Here's how the part is built. I have some questions about the finished solid (model axes, mm). Give positions to 0.01 mm unless a question says otherwise; leave off trailing zeros. Order: outer loops, then holes, each group sorted by start corner. A loop starts at its lowest first (then second) coordinate and runs counter-clockwise, first axis right, second up.
from build123d import *

# Parameters (mm, degrees)
BOSS_EXTRUDE1_DEPTH      = 5
BOSS_EXTRUDE1_DEPTH_BACK = 5
BOSS_EXTRUDE2_DEPTH      = 10
CUT_EXTRUDE1_DEPTH       = 262.627597933
SKETCH4_R                = 1.553741305
CUT_EXTRUDE2_DEPTH       = 215.257438611
CHAMFER1_SIZE            = 2
CHAMFER2_SIZE            = 2
FILLET1_R                = 5


with BuildPart() as part:
    # Sketch1 → Boss-Extrude1 (new, two sides: drawn at the far end of the back side and taken through both)
    with BuildSketch(Plane.XY.offset(-BOSS_EXTRUDE1_DEPTH_BACK)):
        Polygon((-87.5, -200), (-87.5, -40), (-50, 0), (50, 0), (87.5, -40), (87.5, -200), (75.5, -200), (75.5, -44.74536976), (44.80121585, -12), (-44.80121585, -12), (-75.5, -44.74536976), (-75.5, -200), align=None)
    extrude(amount=BOSS_EXTRUDE1_DEPTH + BOSS_EXTRUDE1_DEPTH_BACK)

    # Sketch2 → Boss-Extrude2 (add)
    with BuildSketch(Plane.XY.offset(5)):
        Polygon((-87.5, -200), (-75.5, -200), (-75.5, -197), (-75.5, -157), (-80.5, -157), (-80.5, -195), (-87.5, -195), align=None)
    boss_extrude2 = extrude(amount=BOSS_EXTRUDE2_DEPTH)

    # Sketch3 → Cut-Extrude1 (cut, through all)
    with BuildSketch(Plane.ZY.offset(80.5)):
        Polygon((5, -157), (15, -195), (15, -157), align=None)
    cut_extrude1 = extrude(amount=-CUT_EXTRUDE1_DEPTH, mode=Mode.SUBTRACT)

    # Sketch4 → Cut-Extrude2 (cut, through all)
    with BuildSketch(Plane(origin=(0, -195, 0), x_dir=(1, 0, 0), z_dir=(0, 1, 0))):
        with Locations(Location((-84, -10, 0), (0, 0, 270))):
            Circle(SKETCH4_R)
    cut_extrude2 = extrude(amount=-CUT_EXTRUDE2_DEPTH, mode=Mode.SUBTRACT)

    # Mirror1: Boss-Extrude2, Cut-Extrude1, Cut-Extrude2 across plane
    add(boss_extrude2.mirror(Plane(origin=(0, 0, 0), x_dir=(0, 0, 1), z_dir=(1, 0, 0))))
    add(cut_extrude1.mirror(Plane(origin=(0, 0, 0), x_dir=(0, 0, 1), z_dir=(1, 0, 0))), mode=Mode.SUBTRACT)
    add(cut_extrude2.mirror(Plane(origin=(0, 0, 0), x_dir=(0, 0, 1), z_dir=(1, 0, 0))), mode=Mode.SUBTRACT)

    # Chamfer1
    chamfer1_edges = [part.edges().sort_by_distance(p)[0] for p in [
        (-60.150607925, -28.37268488, -5),
        (0, -12, -5),
        (60.150607925, -28.37268488, -5),
        (75.5, -122.37268488, -5),
        (81.5, -200, -5),
        (87.5, -120, -5),
        (68.75, -20, -5),
        (0, 0, -5),
        (-68.75, -20, -5),
        (-87.5, -120, -5),
        (-81.5, -200, -5),
        (-75.5, -122.37268488, -5),
    ]]
    chamfer(chamfer1_edges, length=CHAMFER1_SIZE)

    # Chamfer2
    chamfer2_edges = [part.edges().sort_by_distance(p)[0] for p in [
        (87.5, -117.5, 5),
        (-60.150607925, -28.37268488, 5),
        (0, -12, 5),
        (60.150607925, -28.37268488, 5),
        (75.5, -100.87268488, 5),
        (68.75, -20, 5),
        (0, 0, 5),
        (-68.75, -20, 5),
        (-87.5, -117.5, 5),
        (-75.5, -100.87268488, 5),
    ]]
    chamfer(chamfer2_edges, length=CHAMFER2_SIZE)

    # Fillet1
    fillet1_edges = [part.edges().sort_by_distance(p)[0] for p in [
        (75.5, -197.5, 15),
        (-75.5, -197.5, 15),
    ]]
    fillet(fillet1_edges, radius=FILLET1_R)


solid = part.part
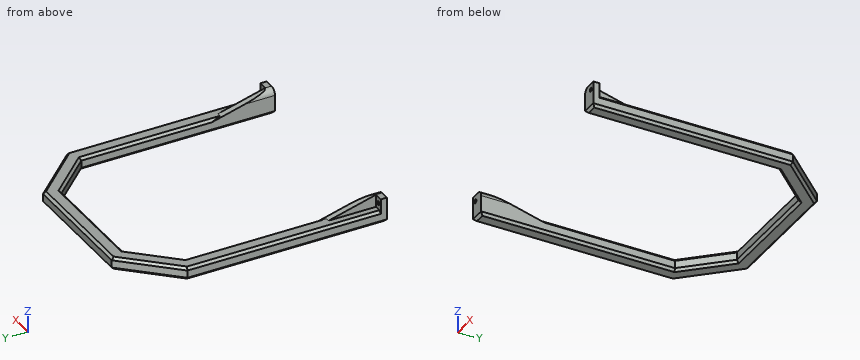
Q1. If we section it at C-C on y = -34: List the corners of the cut face in (x, z) for me (3 decimals).
Filled sheet:
outline: (-81.875, -3) - (-79.134, -5) - (-68.168, -5) - (-65.426, -3) - (-65.426, 3) - (-68.168, 5) - (-79.134, 5) - (-81.875, 3) - close; (65.426, -3) - (68.168, -5) - (79.134, -5) - (81.875, -3) - (81.875, 3) - (79.134, 5) - (68.168, 5) - (65.426, 3) - close
Q2. If we section it at A-A on y = -125.5: List the corners of the cut face in (x, z) for me, plus the area to 3 significant figures.
Filled sheet:
outline: (-87.5, -3) - (-85.5, -5) - (-77.5, -5) - (-75.5, -3) - (-75.5, 3) - (-77.5, 5) - (-85.5, 5) - (-87.5, 3) - close; (75.5, -3) - (77.5, -5) - (85.5, -5) - (87.5, -3) - (87.5, 3) - (85.5, 5) - (77.5, 5) - (75.5, 3) - close
area: 224 mm2
Q3. If we section it at D-D on x = 56: List the corners of the cut face in (y, z) for me, plus the area to 3 significant figures.
Filled sheet:
outline: (-23.95, -3) - (-21.02, -5) - (-9.32, -5) - (-6.4, -3) - (-6.4, 3) - (-9.32, 5) - (-21.02, 5) - (-23.95, 3) - close
area: 164 mm2
Q4. If we section it at B-B on x = -9.5: List the corners of the cut face in (y, z) for me.
Filled sheet:
outline: (-12, -3) - (-10, -5) - (-2, -5) - (0, -3) - (0, 3) - (-2, 5) - (-10, 5) - (-12, 3) - close
Q5. I need wall thicknesses on L1, parallel to X at y = -198.85, z = 10; L2, parallel to Z at x = 84, y = -197; L3, parallel to X at y = -167.5, z = 3. Which ranges of each line are inside material? Lowest first, please.
Filled sheet:
L1: x = -87.5 to -85.55, -82.45 to -75.5, 75.5 to 82.45, 85.55 to 87.5
L2: z = -5 to 8.45, 11.55 to 15
L3: x = -87.5 to -75.5, 75.5 to 87.5
Q6. I'm going to push flat-ended pins straight in: P1, Ø4, axis at y = -100, z = 6, coming from the -X side; P2, Ø7.5, axis at x = -85.5, z = 6, coming from the +Y side; P3, Ø11, axis at y = -171.5, z = 10, coming from the -X side. Where does each tip first touch, or does it pass through?
Filled sheet:
P1: stops at x = -86.5
P2: stops at y = -35.47
P3: stops at x = -86
